Geometry check sheet. Reference: the model listing, model coordinates, mm. A direction names the side the tool comes from. Give positions to 0.01 mm unless a question says otherwise; leave off trailing zeros. Loops run counter-clockwise (first coordinate to the right, second up) from the corner with the lowest first, then second, coordinate; pieces in that order, holes last. Notation, with made-up numbers: (55.25, 29) -> (73.25, 29) arc R8 ccw to (73.25, 38) -> close; hole circle Ø5 at (19, 28). An arc over 180 degrees is marked (long way). One line per item, written item: value. Start each with the question number.
(1) Scan lines: line 1 along X through (y, z) = (49, -14); line 2 along X through (y, z) = (18.5, -12); line 3 along Z through (x, y) = (15, 52). Record each from-to range of solid material in increasing order. Write a range as from..to.
(2) Sectioned sample at C-C, the plane y = 43. Record the cut outline in (x, z), then the cut area to 3 significant figures.
(3) Sectioned sample at A-A, the plane z = 0. Record the cut outline in (x, y).
(4) Draft check along Z on faces 1 (the face through (-3.4, 35, -11)), 2 (the face through (4.336, 34.51, 19.524)), 3 (the face through (6, 0, -1)). Enter one of: pulls with the +Z half, pulls with the -Z half, needs draft (parallel to the pull), parting line crosses it, or undercut.
(5) Sectioned sample at B-B, the plane x = 0. Record the cut outline in (y, z).
(6) Gauge pin test, flat ends, axial feed: pin 1 Ø2.5 at (x, y) = (3, 29) entering from +Z; pin 2 Ø2.5 at (x, y) = (11, 48.5) entering from -Z; pin 3 Ø4 at (x, y) = (0.5, 37.5) entering from -Z. Record the tip position at first contact, or that the pin passes through.
(7) Sectioned sample at D-D, the plane z = 6.5. Record the cut outline in (x, y).
(8) Tool access check on faces 4 (the face through (5.1, 35, 0)), 5 (the face through (6, 70, -1)). Record the directions out of +Z, -Z, +X, -X, +Y, -Y that give a thin tool (end or side, any length) a straight path to the whole face; none if there is none.
Autodesk Inventor part; units mm, degrees
ref_plane "YZ Plane" through (0, 0, 0) normal (1, 0, 0) x (0, 1, 0)
ref_plane "XZ Plane" through (0, 0, 0) normal (0, 1, 0) x (-1, 0, 0)
ref_plane "XY Plane" through (0, 0, 0) normal (0, 0, 1) x (1, 0, 0)
sketch "Sketch1" plane through (0, 0, 0) normal (0, 1, 0) x (-1, 0, 0)
  circle A0 centre (0, 0) radius 20
  line L0 (-8.6, 0) -> (3.4, 0)
  line L1 (3.4, 0) -> (3.4, 7.8994)
  line L2 (3.4, 0) -> (3.4, -7.8994)
  line L3 (3.4, 0) -> (-5.1, 0)
  line L4 (-5.1, 0) -> (-5.1, -4.75)
  line L5 (-5.1, -4.75) -> (3.4, -4.75)
  line L6 (3.4, -4.75) -> (3.4, 0)
  line L7 (-5.1, 0) -> (-5.1, 4.75)
  line L8 (-5.1, 4.75) -> (3.4, 4.75)
  line L9 (-3.1555, 7.8994) -> (-3.1555, 16.1927)
  line L10 (-7.9441, -3.2941) -> (-16.1651, -3.2941)
  line L11 (3.1555, 19.7495) -> (3.4, 19.7495)
  line L12 (-3.1555, -7.8994) -> (-3.1555, -16.1927)
  line L13 (-7.9441, 3.2613) -> (-16.1717, 3.2613)
  line L14 (3.4, 19.7495) -> (3.4, 19.7089)
  line L15 (3.4, 16.1431) -> (3.4, 7.8994)
  line L16 (-8.6, -0.0164) -> (-7.9441, -0.0164)
  line L17 (3.4, -19.7495) -> (3.4, -19.7089)
  line L18 (3.4, -16.1431) -> (3.4, -7.8994)
  arc A1 (-7.9441, -3.2941) -> (-3.1555, -8.0002) centre (0, 0) ccw
  arc A2 (-3.1555, 8.0002) -> (-7.9576, 3.2613) centre (0, 0) ccw
  arc A3 (-8.6, 0) -> (-8.6, -0.0164) centre (0, 0) ccw
  arc A4 (3.4, -16.1431) -> (3.4, 16.1431) centre (0, 0) ccw
  arc A5 (-3.1555, 16.1927) -> (-16.1717, 3.2613) centre (0, 0) ccw
  arc A6 (-16.1651, -3.2941) -> (-3.1555, -16.1927) centre (0, 0) ccw
  point P0 (-3.1555, 19.7495)
  point P1 (-19.7269, -3.2941)
  point P2 (-3.1555, -19.7495)
  point P3 (-19.7269, 3.2613)
  dimension "d0" = 40
  dimension "d2" = 12
  dimension "d4" = 8.5
extrude "Extrusion1" add sketch "Sketch1" along normal blind 70 contours A0
ref_plane "Work Plane1" through (0, 34.925, 0) normal (0, -1, 0) x (1, 0, 0)
equation "\"d6\" = 0.5 * d5"
properties part number "axel"
Calculated:
1. line 1: x = -14.28..-8.73, -3.4..3.16, 8.73..14.28
1. line 2: x = -16..-11.32, -3.4..3.16, 11.32..16
1. line 3: z = -13.23..-6.87, -3.29..3.26, 6.87..13.23
2. outline: circle Ø40 at (0, 0); hole (-3.4, -16.14) -> (-3.4, -4.75) -> (5.1, -4.75) -> (5.1, 4.75) -> (-3.4, 4.75) -> (-3.4, 16.14) arc R16.5 ccw to start; hole (3.16, -16.19) arc R16.5 ccw to (16.17, -3.29) -> (7.94, -3.29) arc R8.6 cw to (3.16, -8) -> close; hole (3.16, 8) arc R8.6 cw to (7.96, 3.26) -> (16.17, 3.26) arc R16.5 ccw to (3.16, 16.19) -> close
2. area: 651 mm2
3. outline: (-20, 0) -> (-16.5, 0) -> (-16.5, 70) -> (-20, 70) -> close; (5.1, 0) -> (20, 0) -> (20, 70) -> (5.1, 70) -> close
4. face 1: undercut
4. face 2: parting line crosses it
4. face 3: needs draft
5. outline: (0, -20) -> (70, -20) -> (70, -4.75) -> (0, -4.75) -> close; (0, 4.75) -> (70, 4.75) -> (70, 20) -> (0, 20) -> close
6. pin 1: stops at z = 19.92
6. pin 2: stops at z = -17.46
6. pin 3: stops at z = -20
7. outline: (-18.91, 0) -> (-15.16, 0) -> (-15.16, 70) -> (-18.91, 70) -> close; (-3.4, 0) -> (5.63, 0) -> (5.63, 70) -> (-3.4, 70) -> close; (15.16, 0) -> (18.91, 0) -> (18.91, 70) -> (15.16, 70) -> close
8. face 4: +Y, -Y
8. face 5: +Z, -Z, +X, -X, +Y
